from build123d import *

# Parameters (mm, degrees)
F0_W     = 40.132
F0_H     = 40.132
F1_DEPTH = 11.6586
F3_DEPTH = 16.51
F4_R     = 9.652
F5_DEPTH = 30.48
F6_R     = 3.175
F7_R     = 3.175
F8_R     = 3.175


with BuildPart() as f1:
    # F0 (on Front) → F1 (new body)
    with BuildSketch(Plane.XZ):
        Rectangle(F0_W, F0_H)
    extrude(amount=F1_DEPTH)

    # F2 (on face) → F3 (join)
    with BuildSketch(Plane.XZ.offset(11.6586)):
        Polygon((-20.066, -9.918316), (-20.066, -20.066), (20.066, -20.066), (20.066, -9.918316), (10.668, 20.066), (-10.668, 20.066), align=None)
    extrude(amount=F3_DEPTH)

    # F4 (on face) → F5 (cut)
    with BuildSketch(Plane(origin=(0, 0, 0), x_dir=(-1, 0, 0), z_dir=(0, 1, 0))):
        Circle(F4_R)
    extrude(amount=-F5_DEPTH, mode=Mode.SUBTRACT)

    # F6
    f6_edges = [f1.edges().sort_by_distance(p)[0] for p in [
        (-20.066, -5.8293, 20.066),
    ]]
    fillet(f6_edges, radius=F6_R)

    # F7
    f7_edges = [f1.edges().sort_by_distance(p)[0] for p in [
        (-20.066, -14.0843, -20.066),
    ]]
    fillet(f7_edges, radius=F7_R)

    # F8
    f8_edges = [f1.edges().sort_by_distance(p)[0] for p in [
        (20.066, -5.8293, 20.066),
        (20.066, -14.0843, -20.066),
    ]]
    fillet(f8_edges, radius=F8_R)


solid = f1.part
CAD build for the part. Positions are in the model's coordinates, mm. A direction names the side the tool comes from. Give positions to 0.01 mm unless a question says otherwise; leave off trailing zeros. Order: outer loops, then holes, each group sorted by start corner. A loop starts at its lowest first (then second) coordinate and runs counter-clockwise, first axis right, second up. Notation, with made-up numbers: (21.25, 65.5) - (44.25, 65.5) arc R17 cw to (44.25, 73.5) - close; hole circle Ø4 at (53, 56.25). An arc over 180 degrees is marked (long way). Answer in a Markdown table with one row per item.
1. Saw through at A-A, the plane x = 0. Give the cut face in (y, z), plus the area to 3 significant figures.
Data:
| item | result |
|---|---|
| outline | (-28.17, -20.07) - (0, -20.07) - (0, -9.65) - (-28.17, -9.65) - close; (-28.17, 9.65) - (0, 9.65) - (0, 20.07) - (-28.17, 20.07) - close |
| area | 587 mm² |
2. Pull direction X, two halves, no side cores. Call faces 4 (the cylindrical face through (19.11, -5.91, 19.16)), 5 (the cylindrical face through (7.66, -13.89, -5.87)), 6 (the flat face through (-5, -28.169, -9)), 7 (the cylindrical face through (-19.16, -5.91, 19.11)): pulls with the +X half, pulls with the -X half, needs draft (parallel to the pull), parting line crosses it, or undercut.
Data:
| item | result |
|---|---|
| face 4 | pulls with the +X half |
| face 5 | undercut |
| face 6 | needs draft |
| face 7 | pulls with the -X half |
3. Probe probe 1 along Z at (x, y) = (0, -20.25); probe 2 along Y at (x, z) = (13.5, 11.5); probe 3 along Z at (x, y) = (-3, -26.25). List the from-to ranges inside material, lowest first. Write a range as [from, to].
Data:
| item | result |
|---|---|
| probe 1 | z = [-20.07, -9.65], [9.65, 20.07] |
| probe 2 | y = [-11.66, 0] |
| probe 3 | z = [-20.07, -9.17], [9.17, 20.07] |
4. Flat gauge pin, fed straight in: pin 1 (8 mm diameter, centred on y = -21, z = -5, fed in from +X). Where does the tip first touch, or does it go through?
Data:
| item | result |
|---|---|
| pin 1 | stops at x = 19.78 |
5. Saw through at B-B, the plane z = -3. Give the cut face in (x, y), plus the area to 3 significant figures.
Data:
| item | result |
|---|---|
| outline | (-20.07, -11.66) - (-17.9, -11.66) - (-17.9, -28.17) - (-9.17, -28.17) - (-9.17, 0) - (-20.07, 0) - close; (9.17, -28.17) - (17.9, -28.17) - (17.9, -11.66) - (20.07, -11.66) - (20.07, 0) - (9.17, 0) - close |
| area | 542 mm² |
6. Saw through at C-C, the plane y = -6.5. Give the cut face in (x, z) (3 decimals), plus the area to 3 significant figures.
Data:
| item | result |
|---|---|
| outline | (-20.066, -16.891) arc R3.175 ccw to (-16.891, -20.066) - (16.891, -20.066) arc R3.175 ccw to (20.066, -16.891) - (20.066, 16.891) arc R3.175 ccw to (16.891, 20.066) - (-16.891, 20.066) arc R3.175 ccw to (-20.066, 16.891) - close; hole circle Ø19.304 at (0, 0) |
| area | 1,310 mm² |
7. Saw through at D-D, the plane z = 4.5. Give the cut face in (x, y), plus the area to 3 significant figures.
Data:
| item | result |
|---|---|
| outline | (-20.07, -11.66) - (-15.55, -11.66) - (-15.55, -28.17) - (-8.54, -28.17) - (-8.54, 0) - (-20.07, 0) - close; (8.54, -28.17) - (15.55, -28.17) - (15.55, -11.66) - (20.07, -11.66) - (20.07, 0) - (8.54, 0) - close |
| area | 500 mm² |
8. Tool access for faces 1 (the flat face through (17, -11.659, 12)), 2 (the flat face through (0, -14, -20.066)), 3 (the flat face through (-16, -11.659, 9)): list every direction of +Z, -Z, +X, -X, +Y, -Y with a clear straight run to the whole face (end or side of a thin tool).
Data:
| item | result |
|---|---|
| face 1 | +Z, +X, -Y |
| face 2 | -Z, +X, -X, +Y, -Y |
| face 3 | +Z, -X, -Y |
